CAD build for the part. Positions are in the model's coordinates, mm. Face numbers are marked on the shaded views. A direction names the side the tool comes from. Give positions to 0.01 mm unless a question says otherwise; leave off trailing zeros. Loops run counter-clockwise (first coordinate to the right, second up) from the corner with the lowest first, then second, coordinate; pieces in that order, holes last.
Item 1: Which spindle directions (+Z, -Z, +X, -X, +Y, -Y) get a long thin tool onto all of the face, cutting with end or side? Do the marked faces 1, 2 and 3. Say none if no direction does.
Item 2: Saw through at B-B on z = 0.75. Give the cut face in (x, y).
Item 3: Saw through at A-A on x = -2. Give the cut face in (y, z).
Item 4: Saw through at D-D on z = -0.5. Give the cut face in (x, y), plus the area to 3 significant figures.
Item 5: Drop flat-ended pins along their axis: P1, Ø2, axis at y = -11, z = 1.5, coming from the +X side; P2, Ø2, axis at y = 3.5, z = 2.5, coming from the +X side; P3, Ø1, axis at x = -5, z = -1, coming from the -Y side; P4, Ø1.5, axis at x = -5, y = -6, coming from the +Z side. Give the stop position or say it passes through.
Item 6: Probe probe 1 along Z at (x, y) = (-4.75, -5); probe 2 along Y at (x, z) = (-4.5, -1.5); probe 3 along Y at (x, z) = (1.75, -0.75). List the from-to ranges inside material, lowest first.
Item 7: Saw through at C-C on x = -5.25. Give the cut face in (y, z), plus the area to 3 significant figures.
Item 8: Mould opens along X. For the marked faces 4, 5 and 6 say: released by +X, released by -X, zero draft, split by the parting line, or undercut.
from build123d import *

# Parameters (mm, degrees)
F1_DEPTH = 2
F4_DEPTH = 11.54701
F5_W     = 7.54701
F5_H     = 6
F6_DEPTH = 25
F8_DEPTH = 7.54701


# Not quite as in the source:
# - the program builds the solid bodies; features that only make, move or delete a surface that nothing else refers to are left out


with BuildPart() as f1:
    # F0 (on Top) → F1 (new body)
    with BuildSketch(Plane.XY):
        Polygon((-3.7735026919, -10), (5.7735026919, -10), (11.5470053838, 0), (5.7735026919, 10), (0, 10), (-5.7735026919, 10), (-11.5470053838, 0), (-6.7735026919, -8.2679491924), (-5.7735026919, -10), align=None)
    extrude(amount=-F1_DEPTH)

    # F3 (on face) → F4 (join)
    with BuildSketch(Plane.YZ.offset(-5.7735026919)):
        Polygon((-10, 2), (-10, 0), (-8, 0), align=None)
        Polygon((-12.2426406871, 2.2426406871), (-10, 0), (-10, 2), (-12.2426406871, 4.2426406871), align=None)
    extrude(amount=F4_DEPTH)

    # F5 (on face) → F6 (cut)
    with BuildSketch(Plane(origin=(0, -4, -4), x_dir=(-1, 0, 0), z_dir=(0, 0.7071067812, 0.7071067812))):
        with Locations((-2.3081e-06, 8.6568542495)):
            Rectangle(F5_W, F5_H)
    extrude(amount=-F6_DEPTH, mode=Mode.SUBTRACT)

    # F7 (on face) → F8 (join, through all)
    with BuildSketch(Plane.YZ.offset(-3.7735026919)):
        Polygon((-12.2426406871, 4.2426406871), (-12.2426406871, 2.2426406871), (-10.2426406871, 2.2426406871), align=None)
    extrude(amount=F8_DEPTH)


solid = f1.part
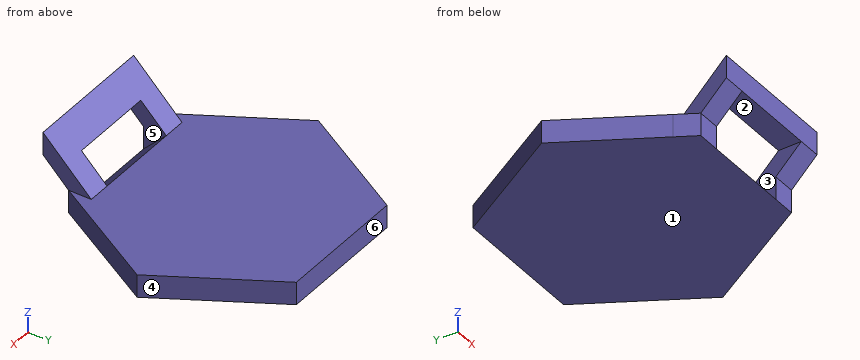
Results below:
1. face 1: -Z, +X, -X, +Y, -Y
1. face 2: -Z, +Y, -Y
1. face 3: -Y
2. outline: (-5.77, -10.75) - (-3.77, -10.75) - (-3.77, -8.75) - (-5.77, -8.75) - close; (3.77, -10.75) - (5.77, -10.75) - (5.77, -8.75) - (3.77, -8.75) - close
3. outline: (-12.24, 2.24) - (-10.24, 2.24) - (-12.24, 4.24) - close; (-10, -2) - (10, -2) - (10, 0) - (-8, 0) - close
4. outline: (-11.55, 0) - (-5.77, -10) - (-3.77, -10) - (-3.77, -8.5) - (3.77, -8.5) - (3.77, -10) - (5.77, -10) - (11.55, 0) - (5.77, 10) - (-5.77, 10) - close
4. area: 335 mm2
5. P1: stops at x = 5.77
5. P2: passes through
5. P3: stops at y = -10
5. P4: stops at z = 0
6. probe 1: z = -2 to 0
6. probe 2: y = -10 to 10
6. probe 3: y = -8.75 to 10
7. outline: (-12.24, 2.24) - (-10, 0) - (-10, -2) - (10, -2) - (10, 0) - (-8, 0) - (-12.24, 4.24) - close
7. area: 46.5 mm2
8. face 4: released by +X
8. face 5: undercut
8. face 6: zero draft
